Could you check a few things on this drawing? It's one solid part, dimensions in mm from its lowest x, y, z. A direction names the side the tool comes from. Coordinates: 2 decimals unless noted, no trailing zeros. Order: outer loops, then holes, each group sorted by start corner. A loop starts at its lowest first (then second) coordinate and runs counter-clockwise, first axis right, second up.
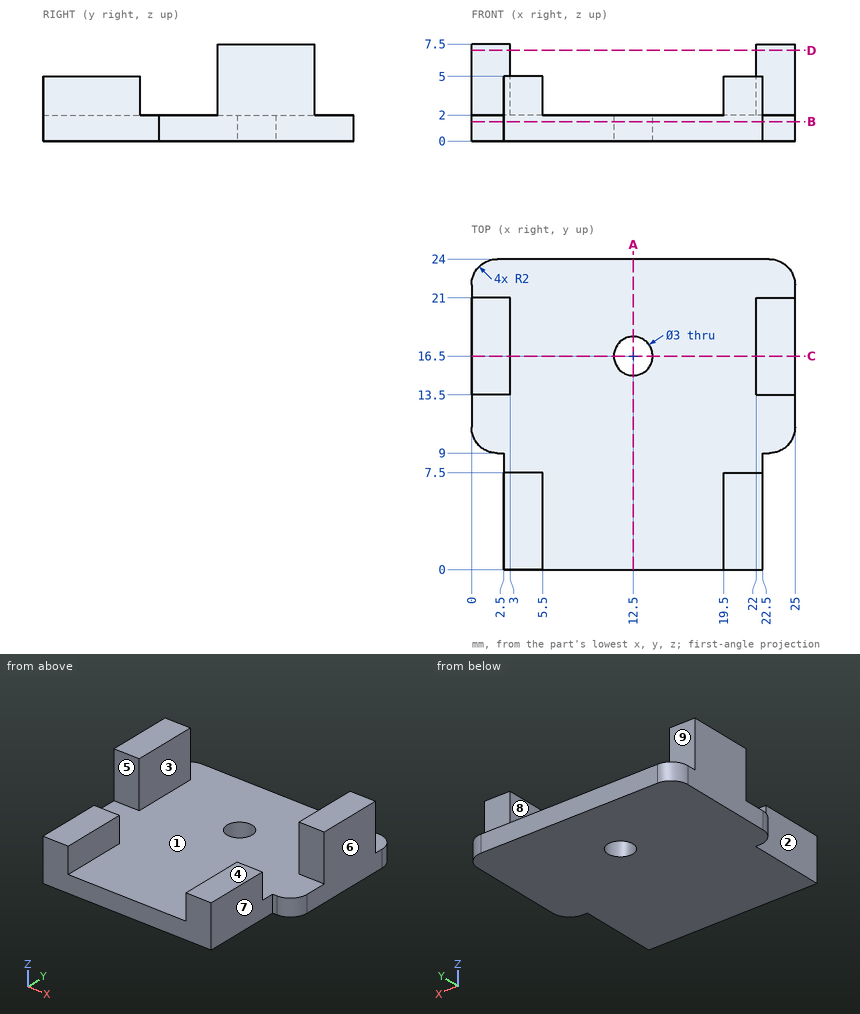
1. Imagine slicing it at B-B on z = 1.5. Please give me the cut outline in (x, y).
Completed:
outline: (0, 11) arc R2 ccw to (2, 9) - (2.5, 9) - (2.5, 0) - (22.5, 0) - (22.5, 9) - (23, 9) arc R2 ccw to (25, 11) - (25, 22) arc R2 ccw to (23, 24) - (2, 24) arc R2 ccw to (0, 22) - close; hole circle Ø3 at (12.5, 16.5)
2. Thinking about a two-plate mould opening in X: for the marked faces 1, 2, 3 and 4, which applies, pulls with the +X half, pulls with the -X half, needs draft (parallel to the pull), parting line crosses it, or undercut?
Completed:
face 1: undercut
face 2: pulls with the -X half
face 3: undercut
face 4: needs draft
3. I'm going to push flat-ended pins straight in: pin 1 (2.5 mm diameter, centred on x = 1.5, z = 6, fed in from -Y); pin 2 (0.9 mm diameter, centred on x = 3.5, y = 4, fed in from +Z); pin 3 (3 mm diameter, centred on x = 5.5, y = 3.5, fed in from -Z); pin 4 (1.5 mm diameter, centred on y = 2.5, z = 2, fed in from -X). Where does each tip first touch, or does it pass through?
Completed:
pin 1: stops at y = 13.5
pin 2: stops at z = 5
pin 3: stops at z = 0
pin 4: stops at x = 2.5
4. Imagine slicing it at D-D on z = 7. Please give me the cut outline in (x, y), then the cut area to 3 significant figures.
Completed:
outline: (0, 13.5) - (3, 13.5) - (3, 21) - (0, 21) - close; (22, 13.5) - (25, 13.5) - (25, 21) - (22, 21) - close
area: 45.0 mm2
5. On a 3-axis mill with a long thin cutter (end or side, diameter ignored), from which of +Z, -Z, +X, -X, +Y, -Y can I reach the whole of each face in a straight line? I mean the marked faces 5, 6, 7, 8 and 9. Say none if no direction works.
Completed:
face 5: +Z, +X, -X
face 6: +Z, -Z, +X, +Y, -Y
face 7: +Z, -Z, +X, -Y
face 8: +Z, +Y
face 9: +Z, +X, -X, +Y
6. Imagine slicing it at C-C on y = 16.5. Please give me the cut outline in (x, z).
Completed:
outline: (0, 0) - (11, 0) - (11, 2) - (3, 2) - (3, 7.5) - (0, 7.5) - close; (14, 0) - (25, 0) - (25, 7.5) - (22, 7.5) - (22, 2) - (14, 2) - close
7. Please list where these lines run through material, in increasing order: probe 1 along Y at (x, z) = (12.5, 1.3); probe 2 along X at (y, z) = (16, 4); probe 3 along Y at (x, z) = (22.25, 2.25).
Completed:
probe 1: y = 0 to 15, 18 to 24
probe 2: x = 0 to 3, 22 to 25
probe 3: y = 0 to 7.5, 13.5 to 21
8. Imagine slicing it at A-A on x = 12.5. Please give me the cut outline in (y, z), then the cut area to 3 significant figures.
Completed:
outline: (0, 0) - (15, 0) - (15, 2) - (0, 2) - close; (18, 0) - (24, 0) - (24, 2) - (18, 2) - close
area: 42.0 mm2
